Geometry check sheet. Reference: the model listing, model coordinates, mm. A direction names the side the tool comes from. Round coordinates to 2 decimals unless told otherwise and drop trailing zeros. Loops run counter-clockwise (first coordinate to the right, second up) from the corner with the lowest first, then second, coordinate; pieces in that order, holes last. Notation, with made-up numbers: M 80,-39.75 L 128,-39.75 A6 cw 128,-34.75 Z; hole C 50.5,6.5 d4. An arc over 180 degrees is marked long. Write item = value, one per line.
from build123d import *

# Parameters (mm, degrees)
SKETCH_2_R      = 12.5
SKETCH_2_R_2    = 11
EXTRUDE_1_DEPTH = 1.5


with BuildPart() as part:
    # 草图1 → 旋转1 (revolve)
    with BuildSketch(Plane.XY, mode=Mode.PRIVATE) as revolve_1_sk:
        Polygon((5, 6), (5, 0), (6.5, 0), (6.5, 0.7), (9.5, 0.7), (9.5, 0), (11, 0), (11, 6), (9.5, 6), (9.5, 5.3), (6.5, 5.3), (6.5, 6), align=None)
    revolve(revolve_1_sk.sketch.rotate(Axis((0, 4.611296038, 0), (0, -1, 0)), 90), axis=Axis((0, 4.611296038, 0), (0, -1, 0)))

    # 草图2 → 凸台-拉伸1 (add)
    with BuildSketch(Plane(origin=(0, 6, 0), x_dir=(1, 0, 0), z_dir=(0, 1, 0))):
        with Locations(Location((0, 0, 0), (0, 0, 270))):
            Circle(SKETCH_2_R)
        with Locations(Location((0, 0, 0), (0, 0, 270))):
            Circle(SKETCH_2_R_2, mode=Mode.SUBTRACT)
    extrude(amount=-EXTRUDE_1_DEPTH)


solid = part.part
(1) Release check for a two-part mould opening along X. For faces 1 (the flat face through (-10, 4.5, 5)), 2 (the cylindrical face through (10.74, 2.28, -2.38)), 3 (the flat face through (6, 0.7, -4)) record: released by +X, released by -X, zero draft, split by the parting line, or undercut.
Result set:
face_1 = zero draft
face_2 = split by the parting line
face_3 = undercut
(2) Material ranges on line 1 along Y through (x, z) = (9.5, -7.5); line 2 along Z through (x, y) = (-3.25, 5.6); line 3 along X through (y, z) = (0.6, 2), recorded low to high. Write a range as from..to.
Result set:
line_1 = 4.5..6
line_2 = -12.07..-8.93, -5.63..-3.8, 3.8..5.63, 8.93..12.07
line_3 = -10.82..-9.29, -6.18..-4.58, 4.58..6.18, 9.29..10.82
(3) Sectioned sample at D-D on z = -7.25. Record the cut outline in (x, y), then the cut area to 3 significant figures.
Result set:
outline = M -10.18,4.5 L -8.27,4.5 L -8.27,0 L -6.14,0 L -6.14,0.7 L 6.14,0.7 L 6.14,0 L 8.27,0 L 8.27,4.5 L 10.18,4.5 L 10.18,6 L 6.14,6 L 6.14,5.3 L -6.14,5.3 L -6.14,6 L -10.18,6 Z
area = 87.8 mm2
(4) Sectioned sample at B-B on x = 0. Record the cut outline in (y, z).
Result set:
outline = M 0,-11 L 4.5,-11 L 4.5,-12.5 L 6,-12.5 L 6,-9.5 L 5.3,-9.5 L 5.3,-6.5 L 6,-6.5 L 6,-5 L 0,-5 L 0,-6.5 L 0.7,-6.5 L 0.7,-9.5 L 0,-9.5 Z; M 0,5 L 6,5 L 6,6.5 L 5.3,6.5 L 5.3,9.5 L 6,9.5 L 6,12.5 L 4.5,12.5 L 4.5,11 L 0,11 L 0,9.5 L 0.7,9.5 L 0.7,6.5 L 0,6.5 Z
(5) Depth check by flat-ended pin: pin 1 Ø1 at (y, z) = (1, 4) entering from +X; pin 2 Ø1 at (y, z) = (3, -9.5) entering from -X; pin 3 Ø2 at (y, z) = (2, -3.5) entering from -X. Enter the tip coordinate at first touch or a pass-through.
Result set:
pin_1 = 10.43
pin_2 = -6.32
pin_3 = -10.71
(6) Sectioned sample at C-C on y = 2.7. Record the cut outline in (x, z).
Result set:
outline = C 0,0 d22; hole C 0,0 d10
(7) Sectioned sample at A-A on z = 0. Record the cut outline in (x, y).
Result set:
outline = M -12.5,4.5 L -11,4.5 L -11,0 L -9.5,0 L -9.5,0.7 L -6.5,0.7 L -6.5,0 L -5,0 L -5,6 L -6.5,6 L -6.5,5.3 L -9.5,5.3 L -9.5,6 L -12.5,6 Z; M 5,0 L 6.5,0 L 6.5,0.7 L 9.5,0.7 L 9.5,0 L 11,0 L 11,4.5 L 12.5,4.5 L 12.5,6 L 9.5,6 L 9.5,5.3 L 6.5,5.3 L 6.5,6 L 5,6 Z
(8) Tool access check on faces 4 (the cylindrical face through (3.955, 0.355, -5.158)), 5 (the flat face through (5, 0, -2)), 6 (the cylindrical face through (3.955, 5.655, -5.158)). Record the directions out of +Z, -Z, +X, -X, +Y, -Y that give a thin tool (end or side, any length) a straight path to the whole face; none if there is none.
Result set:
face_4 = -Y
face_5 = +Z, -Z, +X, -X, -Y
face_6 = +Y
